from build123d import *

# Parameters (mm, degrees)
F0_R     = 17.5
F0_R_2   = 4.75
F0_W     = 6.5
F0_H     = 6.5
F1_DEPTH = 15
F3_R     = 2


# Not quite as in the source:
# - a fillet or chamfer that OpenCascade refuses, or shapes differently, is made with other operations: its cross-section is extruded or revolved along the edge and cut away or added
# - a feature names something its author has since deleted; it is built from what else it names


with BuildPart() as f1:
    # F0 (on Top) → F1 (new body)
    with BuildSketch(Plane.XY):
        Circle(F0_R)
        with Locations((0, -10.2685028687)):
            Circle(F0_R_2, mode=Mode.SUBTRACT)
        Rectangle(F0_W, F0_H, mode=Mode.SUBTRACT)
    extrude(amount=F1_DEPTH)

    # F2: fillet of radius 5 on 2 edges, made by hand

    # F2_s1 → F2_t2 (revolve, cut)
    with BuildSketch(Plane.XZ):
        with BuildLine():
            ThreePointArc((17.5, 10), (16.0355339059, 13.5355339059), (12.5, 15))
            Line((12.5, 15), (17.5, 15))
            Line((17.5, 15), (17.5, 10))
        make_face()
    revolve(axis=Axis((0, 0, 15), (0, 0, 1)), mode=Mode.SUBTRACT)

    # F2_s3 → F2_t4 (revolve, cut)
    with BuildSketch(Plane.XZ):
        with BuildLine():
            ThreePointArc((17.5, 5), (16.0355339059, 1.4644660941), (12.5, 0))
            Line((12.5, 0), (17.5, 0))
            Line((17.5, 0), (17.5, 5))
        make_face()
    revolve(axis=Axis((0, 0, 0), (0, 0, 1)), mode=Mode.SUBTRACT)

    # F3
    f3_edges = [f1.edges().sort_by_distance(p)[0] for p in [
        (-3.25, 0, 15),
        (0, -3.25, 15),
        (0, 3.25, 15),
        (3.25, 0, 15),
        (-3.25, 0, 0),
        (0, -3.25, 0),
        (3.25, 0, 0),
        (0, 3.25, 0),
    ]]
    fillet(f3_edges, radius=F3_R)


solid = f1.part
Input: part model. Units: mm. Frame: model coordinates. A direction names the side the tool comes from. Round coordinates to 2 decimals unless told otherwise and drop trailing zeros. Order: outer loops, then holes, each group sorted by start corner. A loop starts at its lowest first (then second) coordinate and runs counter-clockwise, first axis right, second up. Notation, with made-up numbers: (20, 10.25) - (39, 10.25) arc R28 ccw to (39, 46.25) - close; hole circle Ø8 at (78, 33.5). An arc over 180 degrees is marked (long way). Use a Markdown table: item, result.
1. Section A-A on y = 0. Return the cut outline in (x, z), then the cut area to 3 significant figures.
Evaluation:
| item | result |
|---|---|
| outline | (-17.5, 5) arc R5 ccw to (-12.5, 0) - (-5.25, 0) arc R2 ccw to (-3.25, 2) - (-3.25, 13) arc R2 ccw to (-5.25, 15) - (-12.5, 15) arc R5 ccw to (-17.5, 10) - close; (3.25, 2) arc R2 ccw to (5.25, 0) - (12.5, 0) arc R5 ccw to (17.5, 5) - (17.5, 10) arc R5 ccw to (12.5, 15) - (5.25, 15) arc R2 ccw to (3.25, 13) - close |
| area | 403 mm^2 |
2. Section B-B on x = 0. Return the cut outline in (y, z).
Evaluation:
| item | result |
|---|---|
| outline | (-17.5, 5) arc R5 ccw to (-15.02, 0.68) - (-15.02, 14.32) arc R5 ccw to (-17.5, 10) - close; (-5.52, 0) - (-5.25, 0) arc R2 ccw to (-3.25, 2) - (-3.25, 13) arc R2 ccw to (-5.25, 15) - (-5.52, 15) - close; (3.25, 2) arc R2 ccw to (5.25, 0) - (12.5, 0) arc R5 ccw to (17.5, 5) - (17.5, 10) arc R5 ccw to (12.5, 15) - (5.25, 15) arc R2 ccw to (3.25, 13) - close |
3. Material intervals for probe 1 along Y at (x, z) = (0, 5.5); probe 2 along Y at (x, z) = (1.5, 3.5); probe 3 along X at (y, z) = (-14.5, 12.25), sorted ascending.
Evaluation:
| item | result |
|---|---|
| probe 1 | -17.5 to -15.02, -5.52 to -3.25, 3.25 to 17.5 |
| probe 2 | -17.2 to -14.78, -5.76 to -3.25, 3.25 to 17.2 |
| probe 3 | -8.81 to -2.16, 2.16 to 8.81 |
4. Section C-C on z = 8.5. Return the cut outline in (x, y), then the cut area to 3 significant figures.
Evaluation:
| item | result |
|---|---|
| outline | circle Ø35 at (0, 0); hole circle Ø9.5 at (0, -10.27); hole (-3.25, -3.25) - (3.25, -3.25) - (3.25, 3.25) - (-3.25, 3.25) - close |
| area | 849 mm^2 |
5. Mould query, pull axis Y, two halves, no side actions, for faces 4 (the face through (0.07, 4.12, 0.35)), 5 (the face through (-13.887, -10.648, 7.465)), 6 (the face through (0, 6, 15)). Classes: +Y half, -Y half, draft (parallel to the pull), parting line (faces both ways), or undercut.
Evaluation:
| item | result |
|---|---|
| face 4 | undercut |
| face 5 | parting line |
| face 6 | draft |
6. Access query for faces 1 (the face through (4.12, 0.07, 0.35)), 2 (the face through (4.12, 0.07, 14.65)), 3 (the face through (3.25, 0, 7)). Directions: +Z, -Z, +X, -X, +Y, -Y. A direction counts if a zero-diameter tool reaches every point of the face in a straight line with its end or side. Return the directions, or none.
Evaluation:
| item | result |
|---|---|
| face 1 | -Z |
| face 2 | +Z |
| face 3 | +Z, -Z |
7. First-contact query: pin 1 (7 mm diameter, centred on y = -1, z = 7.5, fed in from +X); pin 2 (5.5 mm diameter, centred on x = 0, y = -10.27, fed in from -Z); pin 3 (3 mm diameter, centred on y = -13, z = 8.5, fed in from -X); pin 4 (3 mm diameter, centred on y = -9.5, z = 3, fed in from -X). Flat tips, straight axial feed; report the tip coordinate or a pass-through.
Evaluation:
| item | result |
|---|---|
| pin 1 | x = 17.5 |
| pin 2 | through |
| pin 3 | x = -13.19 |
| pin 4 | x = -15.28 |
